from build123d import *

# Parameters (mm, degrees)
BOSS_EXTRUDE1_DEPTH = 5.18
CUT_EXTRUDE1_REACH  = 32.745
SKETCH2_W           = 3.45
SKETCH2_H           = 5.15
SKETCH3_W           = 10.5
SKETCH3_H           = 30
SKETCH3_R           = 1.575
BOSS_EXTRUDE2_DEPTH = 1.25
CUT_EXTRUDE3_REACH  = 41.666
SKETCH7_R           = 1.575


with BuildPart() as part:
    # Sketch1 → Boss-Extrude1 (new body)
    with BuildSketch(Plane(origin=(0, 0, 0), x_dir=(0, 0, -1), z_dir=(1, 0, 0))):
        Polygon((0, 0), (13, 0), (13, -7.5), (5.5, -7.5), (5.5, -10.3), (10.25, -10.3), (10.25, -9.8), (5.7, -9.8), (5.7, -7.7), (12.7, -7.7), (12.7, -16.45), (12.9, -16.45), (12.9, -7.7), (15, -7.7), (15, -16.45), (15.5, -16.45), (15.5, -7.7), (17.6, -7.7), (18.85, -17.9), (18.85, -19.15), (0, -19.15), (0, -22.48), (3.25, -22.48), (3.25, -23.73), (-1.25, -23.73), (-1.25, -17.9), (0, -7.7), (2.1, -7.7), (2.1, -16.45), (2.3, -16.45), (2.3, -7.7), (3.3, -7.7), (3.3, -15.15), (8.05, -15.15), (8.05, -14.65), (3.5, -14.65), (3.5, -7.5), (0, -7.5), align=None)
        Polygon((13.7, -8.5), (13.7, -17.7), (1.3, -17.7), (1.3, -8.95), (0.8, -8.95), (0.8, -17.9), (16.8, -17.9), (16.8, -8.95), (16.3, -8.95), (16.3, -17.7), (14.2, -17.7), (14.2, -8.5), align=None, mode=Mode.SUBTRACT)
        Polygon((3.3, -16.45), (11.7, -16.45), (11.7, -8.5), (6.95, -8.5), (6.95, -9), (11.5, -9), (11.5, -13.35), (4.75, -13.35), (4.75, -13.85), (9.3, -13.85), (9.3, -15.95), (3.3, -15.95), align=None, mode=Mode.SUBTRACT)
    extrude(amount=BOSS_EXTRUDE1_DEPTH)

    # Sketch2 → Cut-Extrude1 (cut, up to next)
    with BuildSketch(Plane.XY, mode=Mode.PRIVATE) as cut_extrude1_sk1:
        with Locations((3.455, -3.425)):
            Rectangle(SKETCH2_W, SKETCH2_H)
    cut_extrude1_tool1 = extrude(cut_extrude1_sk1.sketch, amount=-CUT_EXTRUDE1_REACH, mode=Mode.PRIVATE) & part.part
    add(cut_extrude1_tool1.solids().sort_by_distance((3.455, -3.425, 0))[0], mode=Mode.SUBTRACT)

    # Sketch3 → Boss-Extrude2 (add)
    with BuildSketch(Plane.XZ.offset(19.15)):
        with Locations((5.25, -15)):
            Rectangle(SKETCH3_W, SKETCH3_H)
        with Locations(Location((7.62, -15.23, 0), (0, 0, 270))):
            Circle(SKETCH3_R, mode=Mode.SUBTRACT)
        with Locations(Location((7.62, -27.23, 0), (0, 0, 270))):
            Circle(SKETCH3_R, mode=Mode.SUBTRACT)
    extrude(amount=-BOSS_EXTRUDE2_DEPTH)

    # Sketch7 → Cut-Extrude3 (cut, up to next)
    with BuildSketch(Plane.ZY, mode=Mode.PRIVATE) as cut_extrude3_sk1:
        with Locations((-3.25, -3.5)):
            Circle(SKETCH7_R)
    cut_extrude3_tool1 = extrude(cut_extrude3_sk1.sketch, amount=-CUT_EXTRUDE3_REACH, mode=Mode.PRIVATE) & part.part
    # Sketch7 → Cut-Extrude3 (cut, up to next)
    with BuildSketch(Plane.ZY, mode=Mode.PRIVATE) as cut_extrude3_sk2:
        with Locations((-9.75, -3.5)):
            Circle(SKETCH7_R)
    cut_extrude3_tool2 = extrude(cut_extrude3_sk2.sketch, amount=-CUT_EXTRUDE3_REACH, mode=Mode.PRIVATE) & part.part
    add(cut_extrude3_tool1.solids().sort_by_distance((0, -3.5, -3.25))[0], mode=Mode.SUBTRACT)
    add(cut_extrude3_tool2.solids().sort_by_distance((0, -3.5, -9.75))[0], mode=Mode.SUBTRACT)


with BuildPart() as body_2:
    # Mirror3: mirrored copy
    add(part.part.mirror(Plane(origin=(0, 0, 0), x_dir=(0, 0, 1), z_dir=(1, 0, 0))))


solid = body_2.part
Model file for the job. Use its own axes, mm. A direction names the side the tool comes from. Give positions to 0.01 mm unless a question says otherwise; leave off trailing zeros. Write each loop counter-clockwise with the first axis right and the second up, starting at its lowest first coordinate (ties: lowest second). Pieces come first, ordered by that corner, then holes. Notation, with made-up numbers: (36.5, 38.25) -> (55.5, 38.25) arc R19 ccw to (55.5, 75.25) -> close; hole circle Ø9 at (-18, 80.5). An arc over 180 degrees is marked (long way). Write item = value, one per line.
(1) Mould opens along X. For faces 5 (the face through (-5.18, -0.4, -6.6)), 6 (the face through (-8.093, -18.534, -16.732)), 7 (the face through (-3, -11, -3.3)), 8 (the face through (0, -9.4, -7.6)) say: released by +X, released by -X, zero draft, split by the parting line, or undercut.
Determined:
face_5 = released by -X
face_6 = undercut
face_7 = zero draft
face_8 = released by +X
(2) Flat gauge pins, fed straight in: P1, Ø4, axis at x = -3, z = -9, coming from the +Y side; P2, Ø1, axis at x = -2, y = -23, coming from the -Z side; P3, Ø4, axis at x = -3, y = -11.5, coming from the +Z side; P4, Ø2.5, axis at x = -2, y = -12.5, coming from the -Z side. Where does each tip first touch, or does it go through?
Determined:
P1 = 0
P2 = -3.25
P3 = 0.71
P4 = -18.34
(3) Slice it at B-B, the plane z = -27.23. Give the cut face in (x, y) (3 decimals).
Determined:
outline = (-10.5, -19.15) -> (-9.195, -19.15) -> (-9.195, -17.9) -> (-10.5, -17.9) -> close; (-6.045, -19.15) -> (0, -19.15) -> (0, -17.9) -> (-6.045, -17.9) -> close
(4) Probe line 1 along Z through (x, y) = (-7.62, -18.65) (3 decimals); line 2 along Y through (x, z) = (-0.75, -16); line 3 along Z through (x, y) = (-0.5, -2.25). List the from-to ranges inside material, lowest first.
Determined:
line_1 = -30 to -28.805, -25.655 to -16.805, -13.655 to 0
line_2 = -19.15 to -17.9, -17.7 to -7.7
line_3 = -13 to -10.71, -8.79 to -4.21, -2.29 to 0
(5) Tool access for faces 1 (the face through (-3, -12, -15.5)), 2 (the face through (-3, -22.48, -2)), 3 (the face through (-3, -11, -11.5)), 4 (the face through (-3, -7.7, -3)): list every direction of +Z, -Z, +X, -X, +Y, -Y with a clear straight run to the whole face (end or side of a thin tool).
Determined:
face_1 = +X, -X, +Y
face_2 = -Z, +X, -X
face_3 = +X, -X
face_4 = +Z, +X, -X
(6) Slice it at D-D, the plane z = -20.5. Give the cut face in (x, y), then the cut area to 3 significant figures.
Determined:
outline = (-10.5, -19.15) -> (0, -19.15) -> (0, -17.9) -> (-10.5, -17.9) -> close
area = 13.1 mm2
(7) Slice it at A-A, the plane x = -7.62. Give the cut face in (y, z) (3 decimals), then the cut area to 3 significant figures.
Determined:
outline = (-19.15, -30) -> (-17.9, -30) -> (-17.9, -28.805) -> (-19.15, -28.805) -> close; (-19.15, -25.655) -> (-17.9, -25.655) -> (-17.9, -16.805) -> (-19.15, -16.805) -> close; (-19.15, -13.655) -> (-17.9, -13.655) -> (-17.9, 0) -> (-19.15, 0) -> close
area = 29.6 mm2
(8) Slice it at C-C, the plane y = -21. Give the cut face in (x, z).
Determined:
outline = (-5.18, 0) -> (0, 0) -> (0, 1.25) -> (-5.18, 1.25) -> close
